The model under review builds one solid part; all positions refer to its coordinate system, in mm. A direction names the side the tool comes from. Coordinates: 2 decimals unless noted, no trailing zeros. Loops run counter-clockwise (first coordinate to the right, second up) from the corner with the lowest first, then second, coordinate; pieces in that order, holes last. Notation, with made-up numbers: M 1.5,-1.5 L 12.5,-1.5 A13 ccw 12.5,8.5 Z; hole C 0.5,27.5 d2. An arc over 180 degrees is marked long. One line per item, written item: value.
```python
from build123d import *

# Parameters (mm, degrees)
F0_W     = 406.4
F0_H     = 25.4
F0_R     = 3.175
F1_DEPTH = 3.175
F3_DEPTH = 304.8
F4_R     = 3.175
F5_DEPTH = 3.175


# Not quite as in the source:
# - a length typed as a fraction of an inch, garbled in the dataset ("3 / 203.2 mm" for 3/8 in), is restored


with BuildPart() as f1:
    # F0 (on Front) → F1 (new body)
    with BuildSketch(Plane.XZ):
        with Locations((76.9218784556, -2.4463492446)):
            Rectangle(F0_W, F0_H)
        with Locations((-75.4781215444, -2.4463492446)):
            Circle(F0_R, mode=Mode.SUBTRACT)
        with Locations((-24.6781215444, -2.4463492446)):
            Circle(F0_R, mode=Mode.SUBTRACT)
        with Locations((26.1218784556, -2.4463492446)):
            Circle(F0_R, mode=Mode.SUBTRACT)
        with Locations((76.9218784556, -2.4463492446)):
            Circle(F0_R, mode=Mode.SUBTRACT)
        with Locations((127.7218784556, -2.4463492446)):
            Circle(F0_R, mode=Mode.SUBTRACT)
        with Locations((178.5218784556, -2.4463492446)):
            Circle(F0_R, mode=Mode.SUBTRACT)
        with Locations((229.3218784556, -2.4463492446)):
            Circle(F0_R, mode=Mode.SUBTRACT)
    extrude(amount=F1_DEPTH)

    # F2 (on face) → F3 (join)
    with BuildSketch(Plane.XZ.offset(3.175)):
        Polygon((-108.4897565831, 15.5141629976), (-113.7502688252, 10.2536507554), (-109.2601407647, 10.2536507554), (-106.2446925528, 13.2690989673), align=None)
        Polygon((-113.7502688252, 10.2536507554), (-126.2781215444, -2.2742019637), (-126.2781215444, -2.4463492446), (-126.2781215444, -2.6184965255), (-113.7502688252, -15.1463492446), (-109.2601407647, -15.1463492446), (-121.9601407647, -2.4463492446), (-109.2601407647, 10.2536507554), align=None)
        Polygon((-109.2601407647, -15.1463492446), (-113.7502688252, -15.1463492446), (-108.4897565831, -20.4068614867), (-106.2446925528, -18.1617974564), align=None)
    extrude(amount=F3_DEPTH)

    # F4 (on face) → F5 (join)
    with BuildSketch(Plane.XZ.offset(307.975)):
        Polygon((280.1218784556, 10.4257980363), (-109.0879934838, 10.4257980363), (-121.9601407647, -2.4463492446), (-109.4322880456, -14.9742019637), (280.1218784556, -14.9742019637), align=None)
        with Locations((-75.4781215444, -2.4463492446)):
            Circle(F4_R, mode=Mode.SUBTRACT)
        with Locations((-24.6781215444, -2.2742019637)):
            Circle(F4_R, mode=Mode.SUBTRACT)
        with Locations((26.1218784556, -2.2742019637)):
            Circle(F4_R, mode=Mode.SUBTRACT)
        with Locations((76.9218784556, -2.2742019637)):
            Circle(F4_R, mode=Mode.SUBTRACT)
        with Locations((127.7218784556, -2.2742019637)):
            Circle(F4_R, mode=Mode.SUBTRACT)
        with Locations((178.5218784556, -2.2742019637)):
            Circle(F4_R, mode=Mode.SUBTRACT)
        with Locations((229.3218784556, -2.2742019637)):
            Circle(F4_R, mode=Mode.SUBTRACT)
        Polygon((-126.2781215444, 10.4257980363), (-126.2781215444, -2.2742019637), (-113.5781215444, 10.4257980363), align=None)
        Polygon((-113.9224161061, -14.9742019637), (-126.2781215444, -2.6184965255), (-126.2781215444, -14.9742019637), align=None)
        Polygon((-113.5781215444, 10.4257980363), (-126.2781215444, -2.2742019637), (-126.2781215444, -2.6184965255), (-113.9224161061, -14.9742019637), (-109.4322880456, -14.9742019637), (-121.9601407647, -2.4463492446), (-109.0879934838, 10.4257980363), align=None)
    extrude(amount=F5_DEPTH)


solid = f1.part
```
(1) Tool access review of faces 5 (the face through (-114.212, -153.441, 5.301)), 6 (the face through (-123, -3.175, -12)), 7 (the face through (-121, -3.175, 5)): name each direction out of +Z, -Z, +X, -X, +Y, -Y from which nothing blocks a thin tool from reaching the whole face with its end or side.
Checks:
face 5: +X
face 6: -Z, -X
face 7: +Z, -X
(2) To check wall thickness, follow L1, parallel to Y at x = 257, z = 1.5 (3 decimals); L2, parallel to X at y = -104, z = 2; L3, parallel to X at y = -19, z = -4. State the ranges of each line that lie inside material, in increasing order. Write a range as [from, to].
Checks:
L1: [-311.15, -307.975], [-3.175, 0]
L2: [-122, -117.51]
L3: [-124.9, -120.41]
(3) Add section B-B on y = -80. State the section outline as (x, z) points, then the cut area to 3 significant figures.
Checks:
outline: M -126.28,-2.62 L -108.49,-20.41 L -106.24,-18.16 L -121.96,-2.45 L -106.24,13.27 L -108.49,15.51 L -126.28,-2.27 Z
area: 151 mm^2
(4) Insertion check: pin 1 Ø2.5 at (x, y) = (117.5, -1.5) entering from +Z; pin 2 Ø1.6 at (x, z) = (-110.5, -16.5) entering from -Y (3 decimals); pin 3 Ø1.5 at (y, z) = (-112, 7) entering from -X. Each pin has a flat end and moves straight along its axis. Give the tip position at first contact, or say it passes through.
Checks:
pin 1: z = 10.25
pin 2: y = -307.975
pin 3: x = -117.75
(5) Add section A-A on x = 100. State the section outline as (y, z) points (3 decimals).
Checks:
outline: M -311.15,-14.974 L -307.975,-14.974 L -307.975,10.426 L -311.15,10.426 Z; M -3.175,-15.146 L 0,-15.146 L 0,10.254 L -3.175,10.254 Z
(6) Draft analysis for pull direction Y (two halves, no side actions). For faces 1 (the face through (74, -311.15, -5)), 2 (the face through (74, 0, 1)), 3 (the face through (-121, -307.975, 6)), 4 (the face through (76, -3.175, 3)), state which applies: pulls with the +Y half, pulls with the -Y half, needs draft (parallel to the pull), parting line crosses it, or undercut.
Checks:
face 1: pulls with the -Y half
face 2: pulls with the +Y half
face 3: undercut
face 4: undercut
